```python
from build123d import *

# Parameters (mm, degrees)
SKETCH1_W           = 50
SKETCH1_H           = 15
BOSS_EXTRUDE1_DEPTH = 25
SKETCH4_R           = 11.2
CUT_EXTRUDE3_DEPTH  = 58.879184514
SKETCH5_R           = 2.325
SKETCH5_R_2         = 3.35
CUT_EXTRUDE4_DEPTH  = 58.879184514


with BuildPart() as part:
    # Sketch1 → Boss-Extrude1 (new body)
    with BuildSketch(Plane(origin=(0, 0, 0), x_dir=(1, 0, 0), z_dir=(0, 1, 0))):
        with Locations((25, 7.5)):
            Rectangle(SKETCH1_W, SKETCH1_H)
    extrude(amount=BOSS_EXTRUDE1_DEPTH)

    # Sketch4 → Cut-Extrude3 (cut, through all)
    with BuildSketch(Plane(origin=(0, 0, 0), x_dir=(1, 0, 0), z_dir=(0, 1, 0))):
        with Locations((21.42346, 0)):
            Circle(SKETCH4_R)
    extrude(amount=CUT_EXTRUDE3_DEPTH, mode=Mode.SUBTRACT)

    # Sketch5 → Cut-Extrude4 (cut, through all)
    with BuildSketch(Plane.XY):
        with Locations((5.11173, 12.5)):
            Circle(SKETCH5_R)
        with Locations((41.31173, 12.5)):
            Circle(SKETCH5_R_2)
    extrude(amount=-CUT_EXTRUDE4_DEPTH, mode=Mode.SUBTRACT)


solid = part.part
```
Verification items for the finished model (mm, model axes). Round coordinates to 2 decimals unless told otherwise and drop trailing zeros. Order: outer loops, then holes, each group sorted by start corner. A loop starts at its lowest first (then second) coordinate and runs counter-clockwise, first axis right, second up.
1) Material ranges on line 1 (X direction, y = 15.5, z = -6); line 2 (X direction, y = 19.5, z = -6); line 3 (Y direction, x = 41, z = -5.5), recorded low to high.
Geometry says:
line 1: x = 0 to 11.97, 30.88 to 39.82, 42.8 to 50
line 2: x = 0 to 11.97, 30.88 to 50
line 3: y = 0 to 9.16, 15.84 to 25
2) Depth check by flat-ended pin: pin 1 (1.5 mm diameter, centred on x = 19.5, z = -10, fed in from -Y); pin 2 (5 mm diameter, centred on y = 13.5, z = -3.5, fed in from -X). Enter the tip coordinate at first touch or a pass-through.
Geometry says:
pin 1: passes through
pin 2: stops at x = 0
3) Cross-section at A-A, the plane z = -2. Record the cut outline in (x, y) (3 decimals), plus the area to 3 significant figures.
Geometry says:
outline: (0, 0) - (10.403, 0) - (10.403, 25) - (0, 25) - close; (32.443, 0) - (50, 0) - (50, 25) - (32.443, 25) - close; hole circle Ø4.65 at (5.112, 12.5); hole circle Ø6.7 at (41.312, 12.5)
area: 647 mm2
4) Cross-section at D-D, the plane y = 18.5. Record the cut outline in (x, z), plus the area to 3 significant figures.
Geometry says:
outline: (0, -15) - (50, -15) - (50, 0) - (32.62, 0) arc R11.2 cw to (10.22, 0) - (0, 0) - close
area: 553 mm2
5) Draft check along X on faces 1 (the cylindrical face through (38, 13, -7)), 2 (the flat face through (0, 12, -7)), 3 (the flat face through (39.3, 9.5, 0)). Enter one of: +X half, -X half, draft (parallel to the pull), parting line (faces both ways), or undercut.
Geometry says:
face 1: undercut
face 2: -X half
face 3: draft
6) Cross-section at B-B, the plane y = 12.5. Record the cut outline in (x, z).
Geometry says:
outline: (0, -15) - (2.79, -15) - (2.79, 0) - (0, 0) - close; (7.44, -15) - (37.96, -15) - (37.96, 0) - (32.62, 0) arc R11.2 cw to (10.22, 0) - (7.44, 0) - close; (44.66, -15) - (50, -15) - (50, 0) - (44.66, 0) - close
7) Cross-section at C-C, the plane z = -6.25. Record the cut outline in (x, y) (3 decimals).
Geometry says:
outline: (0, 0) - (12.13, 0) - (12.13, 25) - (0, 25) - close; (30.717, 0) - (50, 0) - (50, 25) - (30.717, 25) - close; hole circle Ø4.65 at (5.112, 12.5); hole circle Ø6.7 at (41.312, 12.5)
